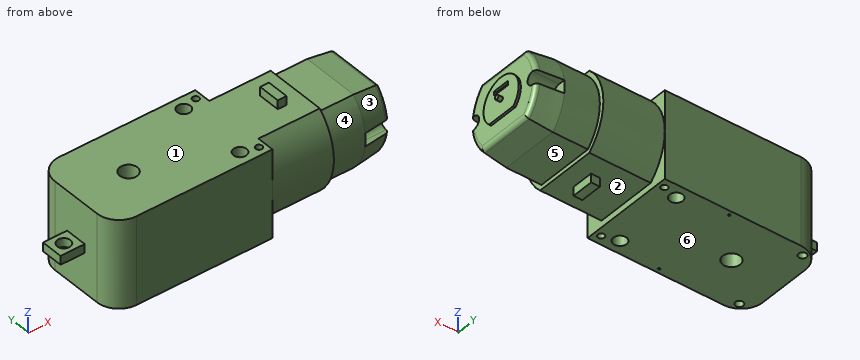
```python
from build123d import *

# Parameters (mm, degrees)
CROQUIS1_W               = 50
CROQUIS1_H               = 20
SALIENTE_EXTRUIR1_DEPTH  = 11
REDONDEO1_R              = 5
CROQUIS2_OUTSIDE_W       = 33.634
CROQUIS2_OUTSIDE_H       = 35.634
CORTAR_EXTRUIR1_DEPTH    = 14
CROQUIS3_R               = 1.5
CORTAR_EXTRUIR2_DEPTH    = 34.85262176
CROQUIS4_W               = 2
CROQUIS4_H               = 5
SALIENTE_EXTRUIR2_DEPTH  = 2
CROQUIS5_W               = 2
CROQUIS5_H               = 5
SALIENTE_EXTRUIR5_DEPTH  = 2
CROQUIS6_R               = 0.75
CROQUIS6_R_2             = 0.25
CROQUIS6_R_3             = 0.9
CORTAR_EXTRUIR3_DEPTH    = 5
CORTAR_EXTRUIR4_START    = -5
CROQUIS7_R               = 0.75
CORTAR_EXTRUIR4_DEPTH    = 5
SALIENTE_EXTRUIR6_DEPTH  = 8
CROQUIS9_R               = 2
CORTAR_EXTRUIR5_DEPTH    = 41.376354466
SALIENTE_EXTRUIR7_DEPTH  = 6
SALIENTE_EXTRUIR7_DRAFT  = 7
REDONDEO2_R              = 1
CROQUIS12_W              = 1
CROQUIS12_H              = 4
SALIENTE_EXTRUIR8_DEPTH  = 0.5
CROQUIS13_R              = 0.5
SALIENTE_EXTRUIR9_DEPTH  = 1
CORTAR_EXTRUIR6_START    = -6
CORTAR_EXTRUIR6_DEPTH    = 6
CROQUIS15_W              = 2
CROQUIS15_H              = 5
SALIENTE_EXTRUIR10_DEPTH = 5.5
CROQUIS16_R              = 1.5
CORTAR_EXTRUIR7_DEPTH    = 44.514365444


with BuildPart() as part:
    # Croquis1 → Saliente-Extruir1 (new, symmetric)
    with BuildSketch(Plane(origin=(0, 0, 0), x_dir=(1, 0, 0), z_dir=(0, 1, 0))):
        Rectangle(CROQUIS1_W, CROQUIS1_H)
    extrude(amount=SALIENTE_EXTRUIR1_DEPTH, both=True)

    # Redondeo1
    redondeo1_edges = [part.edges().sort_by_distance(p)[0] for p in [
        (-25, 11, 0),
        (-25, -11, 0),
    ]]
    fillet(redondeo1_edges, radius=REDONDEO1_R)

    # Croquis2 outside → Cortar-Extruir1 (cut)
    with BuildSketch(Plane(origin=(25, 0, 0), x_dir=(0, 0, -1), z_dir=(1, 0, 0))):
        Rectangle(CROQUIS2_OUTSIDE_W, CROQUIS2_OUTSIDE_H)
        with BuildLine():
            Line((-10, 7), (-10, -7))
            ThreePointArc((-10, -7), (-0.75, -11), (8.5, -7))
            Line((8.5, -7), (8.5, 7))
            ThreePointArc((8.5, 7), (-0.75, 11), (-10, 7))
        make_face(mode=Mode.SUBTRACT)
    extrude(amount=-CORTAR_EXTRUIR1_DEPTH, mode=Mode.SUBTRACT)

    # Croquis3 → Cortar-Extruir2 (cut, through all)
    with BuildSketch(Plane(origin=(0, 0, -10), x_dir=(-1, 0, 0), z_dir=(0, 0, -1))):
        with Locations((-6, 8)):
            Circle(CROQUIS3_R)
        with Locations(Location((-6, -8, 0), (0, 0, 180))):
            Circle(CROQUIS3_R)
    extrude(amount=-CORTAR_EXTRUIR2_DEPTH, mode=Mode.SUBTRACT)

    # Croquis4 → Saliente-Extruir2 (add)
    with BuildSketch(Plane.XY.offset(10)):
        with Locations((20, 0)):
            Rectangle(CROQUIS4_W, CROQUIS4_H)
    extrude(amount=SALIENTE_EXTRUIR2_DEPTH)

    # Croquis5 → Saliente-Extruir5 (add)
    with BuildSketch(Plane(origin=(0, 0, -8.5), x_dir=(-1, 0, 0), z_dir=(0, 0, -1))):
        with Locations((-20, 0)):
            Rectangle(CROQUIS5_W, CROQUIS5_H)
    extrude(amount=SALIENTE_EXTRUIR5_DEPTH)

    # Croquis6 → Cortar-Extruir3 (cut)
    with BuildSketch(Plane(origin=(0, 0, -10), x_dir=(-1, 0, 0), z_dir=(0, 0, -1))):
        with Locations((-9.5, 9)):
            Circle(CROQUIS6_R)
        with Locations((-9.5, -9)):
            Circle(CROQUIS6_R)
        with Locations((4.5, -10)):
            Circle(CROQUIS6_R_2)
        with Locations((4.5, 10)):
            Circle(CROQUIS6_R_2)
        with Locations((22, 9)):
            Circle(CROQUIS6_R_3)
        with Locations((22, -9)):
            Circle(CROQUIS6_R_3)
    extrude(amount=-CORTAR_EXTRUIR3_DEPTH, mode=Mode.SUBTRACT)

    # Croquis7 → Cortar-Extruir4 (cut)
    with BuildSketch(Plane.XY.offset(10).offset(CORTAR_EXTRUIR4_START)):
        with Locations(Location((9.5, -9, 0), (0, 0, 180))):
            Circle(CROQUIS7_R)
        with Locations(Location((9.5, 9, 0), (0, 0, 180))):
            Circle(CROQUIS7_R)
    extrude(amount=CORTAR_EXTRUIR4_DEPTH, mode=Mode.SUBTRACT)

    # Croquis8 → Saliente-Extruir6 (add)
    with BuildSketch(Plane(origin=(25, 0, 0), x_dir=(0, 0, -1), z_dir=(1, 0, 0))):
        with BuildLine():
            Line((-9, 6.594309595), (-9, -6.594309595))
            ThreePointArc((-9, -6.594309595), (-0.75, -10), (7.5, -6.594309595))
            Line((7.5, -6.594309595), (7.5, 6.594309595))
            ThreePointArc((7.5, 6.594309595), (-0.75, 10), (-9, 6.594309595))
        make_face()
    extrude(amount=SALIENTE_EXTRUIR6_DEPTH)

    # Croquis9 → Cortar-Extruir5 (cut, through all)
    with BuildSketch(Plane.XY.offset(10)):
        with Locations((-13, 0)):
            Circle(CROQUIS9_R)
    extrude(amount=-CORTAR_EXTRUIR5_DEPTH, mode=Mode.SUBTRACT)


with BuildPart() as saliente_extruir7_tool:
    # Croquis11 → Saliente-Extruir7 (with draft: the straight prism first)
    with BuildSketch(Plane(origin=(33, 0, 0), x_dir=(0, 0, -1), z_dir=(1, 0, 0))):
        with BuildLine():
            Line((-9, 6.594309595), (-9, -6.594309595))
            ThreePointArc((-9, -6.594309595), (-0.75, -10), (7.5, -6.594309595))
            Line((7.5, -6.594309595), (7.5, 6.594309595))
            ThreePointArc((7.5, 6.594309595), (-0.75, 10), (-9, 6.594309595))
        make_face()
    extrude(amount=SALIENTE_EXTRUIR7_DEPTH)
    # Saliente-Extruir7: the draft: its side faces are tilted about the plane it starts from
    saliente_extruir7_sides = [saliente_extruir7_tool.faces().sort_by_distance(p)[0] for p in [
        (36, 0, 9),
        (36, -10, 0.75),
        (36, 0, -7.5),
        (36, 10, 0.75),
    ]]
    draft(saliente_extruir7_sides, Plane(origin=(33, 0, 0), x_dir=(0, 0, -1), z_dir=(1, 0, 0)), SALIENTE_EXTRUIR7_DRAFT)


with BuildPart() as part_1:
    add(part.part)

    # Saliente-Extruir7: add saliente_extruir7_tool
    add(saliente_extruir7_tool.part)

    # Redondeo2
    redondeo2_edges = [part_1.edges().sort_by_distance(p)[0] for p in [
        (39, 0, -6.763292635),
        (39, -9.263292635, 0.75),
        (39, 0, 8.263292635),
        (39, 9.263292635, 0.75),
    ]]
    fillet(redondeo2_edges, radius=REDONDEO2_R - 0.0001)  # a hair under: the kernel refuses the full size

    # Croquis12 → Saliente-Extruir8 (add)
    with BuildSketch(Plane(origin=(39, 0, 0), x_dir=(0, 0, -1), z_dir=(1, 0, 0))):
        with BuildLine():
            Line((2.87856737, 3.439985297), (2.87856737, -3.439985297))
            ThreePointArc((2.87856737, -3.439985297), (-5.75, 0), (2.87856737, 3.439985297))
        make_face()
        with Locations((-3.25, 0)):
            Rectangle(CROQUIS12_W, CROQUIS12_H, mode=Mode.SUBTRACT)
    extrude(amount=SALIENTE_EXTRUIR8_DEPTH)

    # Croquis13 → Saliente-Extruir9 (add)
    with BuildSketch(Plane(origin=(39.5, 0, 0), x_dir=(0, 0, -1), z_dir=(1, 0, 0))):
        with Locations((-0.75, 0)):
            Circle(CROQUIS13_R)
    extrude(amount=SALIENTE_EXTRUIR9_DEPTH)

    # Croquis14 → Cortar-Extruir6 (cut)
    with BuildSketch(Plane(origin=(39, 0, 0), x_dir=(0, 0, -1), z_dir=(1, 0, 0)).offset(CORTAR_EXTRUIR6_START)):
        with BuildLine():
            Line((-2.25, 9.903408743), (-2.25, 8.403408743))
            ThreePointArc((-2.25, 8.403408743), (-0.75, 6.903408743), (0.75, 8.403408743))
            Line((0.75, 8.403408743), (0.75, 9.903408743))
            ThreePointArc((0.75, 9.903408743), (-0.75, 10), (-2.25, 9.903408743))
        make_face()
        with BuildLine():
            Line((-2.25, -9.903408743), (-2.25, -8.403408743))
            ThreePointArc((-2.25, -8.403408743), (-0.75, -6.903408743), (0.75, -8.403408743))
            Line((0.75, -8.403408743), (0.75, -9.903408743))
            ThreePointArc((0.75, -9.903408743), (-0.75, -10), (-2.25, -9.903408743))
        make_face()
    extrude(amount=CORTAR_EXTRUIR6_DEPTH, mode=Mode.SUBTRACT)

    # Croquis15 → Saliente-Extruir10 (add)
    with BuildSketch(Plane.ZY.offset(25)):
        Rectangle(CROQUIS15_W, CROQUIS15_H)
    extrude(amount=SALIENTE_EXTRUIR10_DEPTH)

    # Croquis16 → Cortar-Extruir7 (cut, through all)
    with BuildSketch(Plane.XY.offset(1)):
        with Locations((-27.75, 0)):
            Circle(CROQUIS16_R)
    extrude(amount=-CORTAR_EXTRUIR7_DEPTH, mode=Mode.SUBTRACT)


solid = part_1.part
```
Source: CAD feature listing. Evaluate the final solid. Frame: model axes, mm. Face numbers are marked on the shaded views. A direction names the side the tool comes from. Give positions to 0.01 mm unless a question says otherwise; leave off trailing zeros. Order: outer loops, then holes, each group sorted by start corner. A loop starts at its lowest first (then second) coordinate and runs counter-clockwise, first axis right, second up.
(1) Material intervals for line 1 along Y through (x, z) = (-4.5, -6.9); line 2 along Y through (x, z) = (6, -3.75); line 3 along X through (y, z) = (5.5, -5.75), sorted ascending.
(2) Contact query for flat-ended pins moving along their axis: P1, Ø1.2, axis at x = 9.5, y = 9, coming from the -Z side; P2, Ø1.5, axis at x = -17, y = -6, coming from the -Z side; P3, Ø5, axis at x = -11.5, y = -1, coming from the +Z side; P4, Ø1, axis at x = -12.5, y = 0.5, coming from the -Z side. Output: stop coordinate, or through.
(3) Pull-direction query (X, two-part tool) for the marked faces 1, 2 and 3; classes: +X half, -X half, draft (parallel to the pull), parting line (faces both ways), or undercut.
(4) Section query D-D (x = 34.5). Return the cut outline in (y, z), plus the area to 3 significant figures.
(5) Access query for the marked faces 4, 5 and 6. Directions: +Z, -Z, +X, -X, +Y, -Y. A direction counts if a zero-diameter tool reaches every point of the face in a straight line with its end or side. Return the directions, or none.
(6) Section query B-B (x = 9.5). Return the cut outline in (y, z), plus the area to 3 significant figures.
(7) Section query C-C (y = 4.25). Return the cut outline in (x, z), plus the area to 3 significant figures.
(8) Section query A-A (x = -27.75). Return the cut outline in (y, z).
Outcome:
1. line 1: y = -11 to -10.25, -9.75 to 9.75, 10.25 to 11
1. line 2: y = -11 to -9.5, -6.5 to 6.5, 9.5 to 11
1. line 3: x = -25 to 39
2. P1: stops at z = -5
2. P2: stops at z = -10
2. P3: stops at z = 10
2. P4: passes through
3. face 1: draft
3. face 2: undercut
3. face 3: +X half
4. outline: (-9.72, -0.75) arc R11.51 ccw to (-6.52, -7.32) - (6.52, -7.32) arc R11.51 ccw to (9.72, -0.75) - (8.4, -0.75) arc R1.5 cw to (8.4, 2.25) - (9.72, 2.25) arc R11.51 ccw to (6.52, 8.82) - (-6.52, 8.82) arc R11.51 ccw to (-9.72, 2.25) - (-8.4, 2.25) arc R1.5 cw to (-8.4, -0.75) - close
4. area: 268 mm2
5. face 4: +X, -Y
5. face 5: -Z, +X, +Y, -Y
5. face 6: -Z, -X, +Y, -Y
6. outline: (-11, -10) - (-9.75, -10) - (-9.75, -5) - (-8.25, -5) - (-8.25, -10) - (8.25, -10) - (8.25, -5) - (9.75, -5) - (9.75, -10) - (11, -10) - (11, 10) - (9.75, 10) - (9.75, 5) - (8.25, 5) - (8.25, 10) - (-8.25, 10) - (-8.25, 5) - (-9.75, 5) - (-9.75, 10) - (-11, 10) - close
6. area: 410 mm2
7. outline: (-25, -10) - (11, -10) - (11, -8.5) - (25, -8.5) - (25, -7.5) - (33, -7.5) - (38.12, -6.87) arc R1 ccw to (39, -5.88) - (39, -1.88) - (39.5, -1.88) - (39.5, 3.38) - (39, 3.38) - (39, 7.38) arc R1 ccw to (38.12, 8.37) - (33, 9) - (25, 9) - (25, 10) - (-25, 10) - close
7. area: 1,210 mm2
8. outline: (-2.5, -1) - (-1.5, -1) - (-1.5, 1) - (-2.5, 1) - close; (1.5, -1) - (2.5, -1) - (2.5, 1) - (1.5, 1) - close
